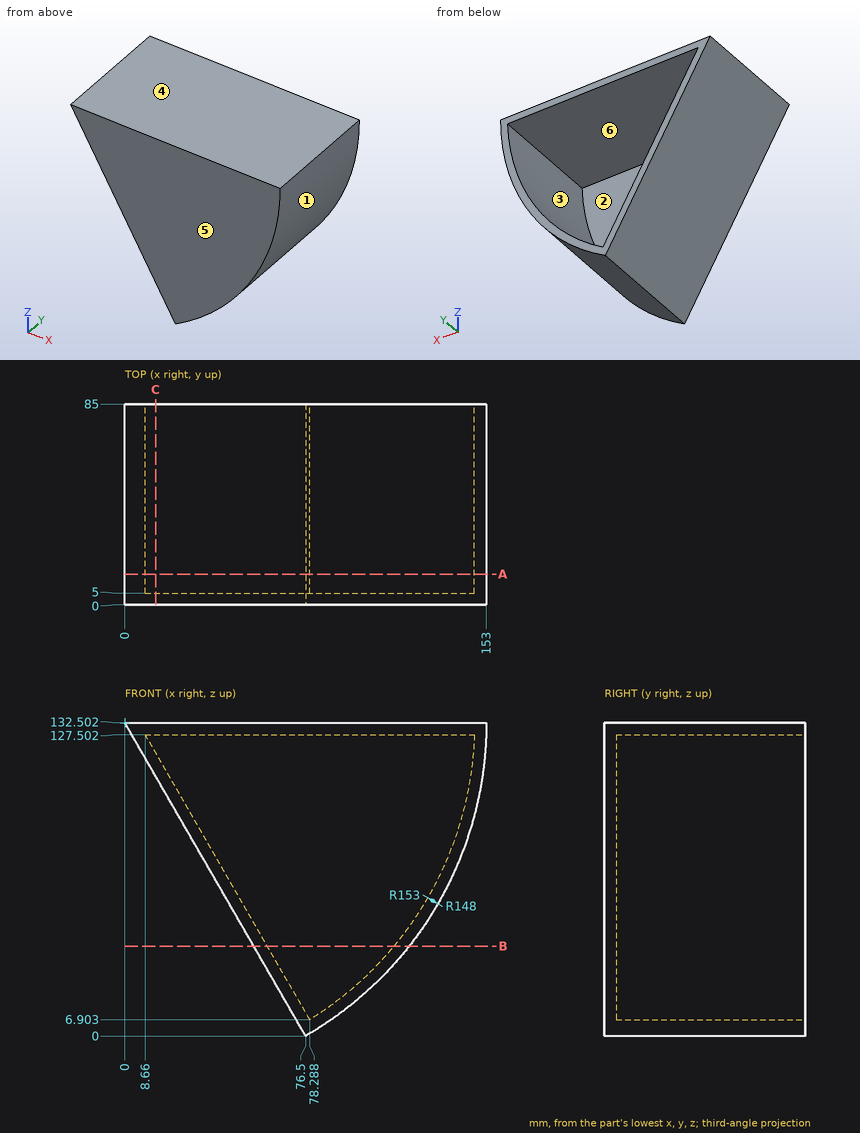
Here's the drawing with two shaded views (mm, measured from the low corner). I have some questions. A direction names the side the tool comes from. Round coordinates to 2 decimals unless told otherwise and drop trailing zeros. Loops run counter-clockwise (first coordinate to the right, second up) from the corner with the lowest first, then second, coordinate; pieces in that order, holes last.
Item 1: Which directions (+Z, -Z, +X, -X, +Y, -Y) give clear straight access to the entire face, cutting with the end or side of a thin tool? Please do the marked faces 5 and 6.
Item 2: If we mould it in two halves opening along Z, with no side actions, what happens to the marked faces 1, 2, 3 and 4? For each: +Z half, -Z half, draft (parallel to the pull), parting line (faces both ways), or undercut.
Item 3: Suppose I cut it at C-C, the plane x = 13. Write out the boundary of the cut face in (y, z) (1 decimal), then the cut area to 3 significant figures.
Item 4: Please list where these lines run through material, in increasing order: L1, parallel to Y at x = 83.5, z = 36; L2, parallel to Z at x = 43, y = 81 (1 decimal); L3, parallel to X at y = 37.5, z = 65 (1 decimal).
Item 5: Suppose I cut it at A-A, the plane y = 13. Write out the boundary of the cut face in (x, z) (1 decimal), then the cut area to 3 significant figures.
Item 6: Will these pins go through, and if not, where does the flat tip stop? pin 1 Ø10 at (y, z) = (74, 94.5) entering from -X; pin 2 Ø1.5 at (y, z) = (32, 15) entering from +X (1 decimal); pin 3 Ø8 at (y, z) = (53.5, 15) entering from -X.
Item 7: Suppose I cut it at B-B, the plane z = 38. Write out the boundary of the cut face in (x, y).
Reported:
1. face 5: +Z, -Z, +X, -X, -Y
1. face 6: +Y
2. face 1: -Z half
2. face 2: undercut
2. face 3: undercut
2. face 4: +Z half
3. outline: (0, 110) - (85, 110) - (85, 120) - (5, 120) - (5, 127.5) - (85, 127.5) - (85, 132.5) - (0, 132.5) - close
3. area: 1,310 mm2
4. L1: y = 0 to 5
4. L2: z = 58 to 68, 127.5 to 132.5
4. L3: x = 39 to 44.7, 131.7 to 137.3
5. outline: (0, 132.5) - (76.5, 0) arc R153 ccw to (153, 132.5) - close; hole (8.7, 127.5) - (78.3, 6.9) arc R148 ccw to (147.9, 127.5) - close
5. area: 2,220 mm2
6. pin 1: stops at x = 19.05
6. pin 2: stops at x = 98.9
6. pin 3: stops at x = 65.53
7. outline: (54.56, 0) - (120.33, 0) - (120.33, 85) - (113.9, 85) - (113.9, 5) - (60.33, 5) - (60.33, 85) - (54.56, 85) - close
